from build123d import *

# Parameters (mm, degrees)
F1_DEPTH = 15.875


with BuildPart() as f1:
    # F0 (on Front) → F1 (new body)
    with BuildSketch(Plane.XZ):
        with BuildLine():
            Line((702.561291, 25.4), (-59.438709, 25.4))
            Line((-59.438709, 25.4), (-59.438709, 0))
            ThreePointArc((-59.438709, 0), (-29.659824, -145.080478), (54.861291, -266.7))
            ThreePointArc((54.861291, -266.7), (82.960432, -412.500368), (169.161291, -533.4))
            Line((169.161291, -533.4), (702.561291, -533.4))
            Line((702.561291, -533.4), (702.561291, 25.4))
        make_face()
    extrude(amount=F1_DEPTH)


solid = f1.part
Could you check a few things on this model? Use its own coordinates, in mm. Round coordinates to 2 decimals unless told otherwise and drop trailing zeros. Write each loop counter-clockwise with the first axis right and the second up, starting at its lowest first coordinate (ties: lowest second). Pieces come first, ordered by that corner, then holes. Notation, with made-up numbers: (18, -39.75) -> (43, -39.75) arc R16 ccw to (43, -31.75) -> close; hole circle Ø2 at (-24.75, -6.75). An arc over 180 degrees is marked (long way). Use a Markdown table: item, result.
1. Please list where these lines run through material, in increasing order: probe 1 along X at (y, z) = (-12, -274); probe 2 along X at (y, z) = (-5.5, -23); probe 3 along Z at (x, y) = (86, -14.5).
Answer key:
| item | result |
|---|---|
| probe 1 | x = 54.76 to 702.56 |
| probe 2 | x = -58.72 to 702.56 |
| probe 3 | z = -419.39 to 25.4 |
2. For pin 1 Ø4 at (x, y) = (89.5, -2) entering from -Z; pin 2 Ø6 at (y, z) = (-4, -447.5) entering from -X, each with a flat end and sliding along its axis, tell me the tip position at first contact or that it passes through.
Answer key:
| item | result |
|---|---|
| pin 1 | stops at z = -430.93 |
| pin 2 | stops at x = 98.66 |
3. If we section it at C-C (x = 23.5): List the corners of the cut face in (y, z) for me (3 decimals).
Answer key:
| item | result |
|---|---|
| outline | (-15.875, -232.839) -> (0, -232.839) -> (0, 25.4) -> (-15.875, 25.4) -> close |
4. If we section it at B-B (z = -410): List the corners of the cut face in (x, y) for me (3 decimals).
Answer key:
| item | result |
|---|---|
| outline | (81.9, -15.875) -> (702.561, -15.875) -> (702.561, 0) -> (81.9, 0) -> close |
5. If we section it at A-A (y = -5.25): List the corners of the cut face in (x, z) for me.
Answer key:
| item | result |
|---|---|
| outline | (-59.44, 0) arc R368.3 ccw to (54.86, -266.7) arc R348.78 ccw to (169.16, -533.4) -> (702.56, -533.4) -> (702.56, 25.4) -> (-59.44, 25.4) -> close |
